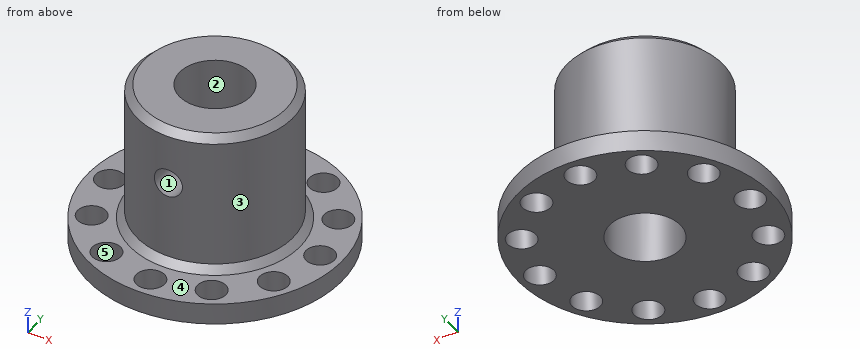
```python
from build123d import *

# Parameters (mm, degrees)
SKETCH1_R           = 17.904347826
BOSS_EXTRUDE1_DEPTH = 3
SKETCH2_R           = 11
BOSS_EXTRUDE2_DEPTH = 20
SKETCH3_R           = 5
CUT_EXTRUDE1_DEPTH  = 24
SKETCH4_R           = 2
CUT_EXTRUDE2_DEPTH  = 15
CHAMFER1_SIZE       = 1
SKETCH5_R           = 2
CUT_EXTRUDE5_DEPTH  = 4.0000001
CIRPATTERN2_COUNT   = 12
SCALE1_SCALE        = 0.630434783


with BuildPart() as part:
    # Sketch1 → Boss-Extrude1 (new body)
    with BuildSketch(Plane.XY):
        Circle(SKETCH1_R)
    extrude(amount=BOSS_EXTRUDE1_DEPTH)

    # Sketch2 → Boss-Extrude2 (add)
    with BuildSketch(Plane.XY.offset(3)):
        Circle(SKETCH2_R)
    extrude(amount=BOSS_EXTRUDE2_DEPTH)

    # Sketch3 → Cut-Extrude1 (cut, through all)
    with BuildSketch(Plane.XY.offset(23)):
        Circle(SKETCH3_R)
    extrude(amount=-CUT_EXTRUDE1_DEPTH, mode=Mode.SUBTRACT)

    # Sketch4 → Cut-Extrude2 (cut)
    with BuildSketch(Plane(origin=(0, 0, 0), x_dir=(1, 0, 0), z_dir=(0, 1, 0))):
        with Locations((0, -15)):
            Circle(SKETCH4_R)
    extrude(amount=-CUT_EXTRUDE2_DEPTH, mode=Mode.SUBTRACT)

    # Chamfer1
    chamfer1_edges = [part.edges().sort_by_distance(p)[0] for p in [
        (-11, 0, 3),
        (-11, 0, 23),
    ]]
    chamfer(chamfer1_edges, length=CHAMFER1_SIZE)

    # Sketch5 → Cut-Extrude5 (cut, through all)
    with BuildSketch(Plane.XY.offset(3)):
        with Locations((7.502173913, 12.994146385)):
            Circle(SKETCH5_R)
    cut_extrude5 = extrude(amount=-CUT_EXTRUDE5_DEPTH, mode=Mode.SUBTRACT)

    # CirPattern2: Cut-Extrude5 ×12 about axis
    cirpattern2_axis = Axis((0, 0, 0), (0, 0, 1))
    for i in range(1, CIRPATTERN2_COUNT):
        add(cut_extrude5.rotate(cirpattern2_axis, i * 360 / CIRPATTERN2_COUNT), mode=Mode.SUBTRACT)


with BuildPart() as part_1:
    # Scale1: scaled about (0, 0, 0)
    add(part.part.scale(SCALE1_SCALE))


solid = part_1.part
```
Verification items for the finished model (mm, model axes). Face numbers are marked on the shaded views. A direction names the side the tool comes from. Coordinates: 2 decimals unless noted, no trailing zeros. Loops run counter-clockwise (first coordinate to the right, second up) from the corner with the lowest first, then second, coordinate; pieces in that order, holes last. Notation, with made-up numbers: (66, -25) - (112, -25) arc R21 ccw to (112, 1) - close; hole circle Ø6 at (58.5, 52.5). An arc over 180 degrees is marked (long way). Return JSON: item names as keys, results as strings.
1. Section check A-A, the plane y = 0. Record the boundary of the cut face in (x, z).
Established:
{"outline": "(-11.29, 0) - (-10.72, 0) - (-10.72, 1.89) - (-11.29, 1.89) - close; (-8.2, 0) - (-3.15, 0) - (-3.15, 14.5) - (-6.3, 14.5) - (-6.93, 13.87) - (-6.93, 2.52) - (-7.57, 1.89) - (-8.2, 1.89) - close; (3.15, 0) - (8.2, 0) - (8.2, 1.89) - (7.57, 1.89) - (6.93, 2.52) - (6.93, 13.87) - (6.3, 14.5) - (3.15, 14.5) - close; (10.72, 0) - (11.29, 0) - (11.29, 1.89) - (10.72, 1.89) - close"}
2. Mould release check, pull along Y, two halves, no side actions. Record for the marked faces 3, 4 and 5: +Y half, -Y half, draft (parallel to the pull), parting line (faces both ways), or undercut.
Established:
{"face 3": "parting line", "face 4": "draft", "face 5": "undercut"}
3. Thickness scan on L1, parallel to X at y = -4.5, z = 0.5; L2, parallel to X at y = 9.25, z = 1; L3, parallel to X at y = 1, z = 10. Record the ranges inside material, lowest first.
Established:
{"L1": "x = -10.35 to -9.43, -6.95 to 6.95, 9.43 to 10.35", "L2": "x = -6.47 to -5.42, -4.04 to -1.24, 1.24 to 4.04, 5.42 to 6.47", "L3": "x = -6.86 to -2.99, 2.99 to 6.86"}
4. Section check C-C, the plane x = -8.5. Record the boundary of the cut face in (y, z), then the cut area to 3 significant figures.
Established:
{"outline": "(-7.43, 0) - (-5.95, 0) - (-5.95, 1.89) - (-7.43, 1.89) - close; (-3.51, 0) - (-0.82, 0) - (-0.82, 1.89) - (-3.51, 1.89) - close; (0.82, 0) - (3.51, 0) - (3.51, 1.89) - (0.82, 1.89) - close; (5.95, 0) - (7.43, 0) - (7.43, 1.89) - (5.95, 1.89) - close", "area": "15.7 mm2"}
5. Go/stop test with flat-tipped pins: pin 1 (3.5 mm diameter, centred on x = 9.46, y = 0, fed in from -Z); pin 2 (2 mm diameter, centred on x = 2.5, z = 3.5, fed in from -Y); pin 3 (1.5 mm diameter, centred on x = -9.46, y = 0, fed in from -Z); pin 4 (4 mm diameter, centred on x = -4.73, y = -8.19, fed in from +Z). Record where each tip stops, or that it passes through.
Established:
{"pin 1": "stops at z = 0", "pin 2": "stops at y = -6.77", "pin 3": "passes through", "pin 4": "stops at z = 2"}
6. Section check D-D, the plane z = 4.75. Record the boundary of the cut face in (x, y), then the cut area to 3 significant figures.
Established:
{"outline": "circle Ø13.87 at (0, 0); hole circle Ø6.3 at (0, 0)", "area": "120 mm2"}
7. Section check B-B, the plane x = 0. Record the boundary of the cut face in (y, z).
Established:
{"outline": "(-11.29, 0) - (-10.72, 0) - (-10.72, 1.89) - (-11.29, 1.89) - close; (-8.2, 0) - (-3.15, 0) - (-3.15, 8.2) - (-6.93, 8.2) - (-6.93, 2.52) - (-7.57, 1.89) - (-8.2, 1.89) - close; (-6.93, 10.72) - (-3.15, 10.72) - (-3.15, 14.5) - (-6.3, 14.5) - (-6.93, 13.87) - close; (3.15, 0) - (8.2, 0) - (8.2, 1.89) - (7.57, 1.89) - (6.93, 2.52) - (6.93, 13.87) - (6.3, 14.5) - (3.15, 14.5) - close; (10.72, 0) - (11.29, 0) - (11.29, 1.89) - (10.72, 1.89) - close"}
8. Tool access check on the marked faces 1 and 2. Record the directions out of +Z, -Z, +X, -X, +Y, -Y that give a thin tool (end or side, any length) a straight path to the whole face; none if there is none.
Established:
{"face 1": "-Y", "face 2": "+Z, -Z"}
